```python
from build123d import *

# Parameters (mm, degrees)
CROQUIS1_R              = 3.25
CROQUIS1_R_2            = 2.25
SALIENTE_EXTRUIR1_DEPTH = 10
SALIENTE_EXTRUIR2_DEPTH = 10
CROQUIS3_R              = 2.25
CORTAR_EXTRUIR1_DEPTH   = 128.867118525
CROQUIS4_R              = 10.9
CORTAR_EXTRUIR2_DEPTH   = 7
CROQUIS5_R              = 4.25
CORTAR_EXTRUIR3_DEPTH   = 128.667536986
CROQUIS6_R              = 2.5
CORTAR_EXTRUIR4_DEPTH   = 128.867118525


with BuildPart() as part:
    # Croquis1 → Saliente-Extruir1 (new body)
    with BuildSketch(Plane(origin=(0, 0, 0), x_dir=(0, 0, -1), z_dir=(1, 0, 0))):
        with BuildLine():
            Line((-25, 0), (-25, -85))
            Line((-25, -85), (25, -85))
            Line((25, -85), (25, 0))
            ThreePointArc((25, 0), (0, 25), (-25, 0))
        make_face()
        Circle(CROQUIS1_R, mode=Mode.SUBTRACT)
        with Locations((-8, 8)):
            Circle(CROQUIS1_R_2, mode=Mode.SUBTRACT)
        with Locations((8, 8)):
            Circle(CROQUIS1_R_2, mode=Mode.SUBTRACT)
        with Locations((8, -8)):
            Circle(CROQUIS1_R_2, mode=Mode.SUBTRACT)
        with Locations((-8, -8)):
            Circle(CROQUIS1_R_2, mode=Mode.SUBTRACT)
    extrude(amount=SALIENTE_EXTRUIR1_DEPTH)

    # Croquis2 → Saliente-Extruir2 (add)
    with BuildSketch(Plane(origin=(10, 0, 0), x_dir=(0, 0, -1), z_dir=(1, 0, 0))):
        with BuildLine():
            Line((-25, -100), (-25, -85))
            Line((-25, -85), (25, -85))
            Line((25, -85), (25, -100))
            ThreePointArc((25, -100), (0, -125), (-25, -100))
        make_face()
    extrude(amount=-SALIENTE_EXTRUIR2_DEPTH)

    # Croquis3 → Cortar-Extruir1 (cut, through all)
    with BuildSketch(Plane.ZY):
        with Locations((0, -35)):
            Circle(CROQUIS3_R)
        with Locations((0, -65)):
            Circle(CROQUIS3_R)
    extrude(amount=-CORTAR_EXTRUIR1_DEPTH, mode=Mode.SUBTRACT)

    # Croquis4 → Cortar-Extruir2 (cut)
    with BuildSketch(Plane.ZY):
        with Locations((0, -100)):
            Circle(CROQUIS4_R)
    extrude(amount=-CORTAR_EXTRUIR2_DEPTH, mode=Mode.SUBTRACT)

    # Croquis5 → Cortar-Extruir3 (cut, through all)
    with BuildSketch(Plane.ZY.offset(-7)):
        with Locations((0, -100)):
            Circle(CROQUIS5_R)
    extrude(amount=-CORTAR_EXTRUIR3_DEPTH, mode=Mode.SUBTRACT)

    # Croquis6 → Cortar-Extruir4 (cut, through all)
    with BuildSketch(Plane.ZY):
        with Locations((17.95, -100)):
            Circle(CROQUIS6_R)
    extrude(amount=-CORTAR_EXTRUIR4_DEPTH, mode=Mode.SUBTRACT)


solid = part.part
```
Source: CAD feature listing. Evaluate the final solid. Frame: model axes, mm. A direction names the side the tool comes from. Give positions to 0.01 mm unless a question says otherwise; leave off trailing zeros. Order: outer loops, then holes, each group sorted by start corner. A loop starts at its lowest first (then second) coordinate and runs counter-clockwise, first axis right, second up. Notation, with made-up numbers: (36, -4) -> (90, -4) arc R12 ccw to (90, 2) -> close; hole circle Ø2 at (63.5, 58). An arc over 180 degrees is marked (long way). Use a Markdown table: item, result.
Q1. Section D-D (z = 17.95). Return the cut outline in (x, y).
A:
| item | result |
|---|---|
| outline | (0, -117.4) -> (10, -117.4) -> (10, -102.5) -> (0, -102.5) -> close; (0, -97.5) -> (10, -97.5) -> (10, 17.4) -> (0, 17.4) -> close |
Q2. Pull-direction query (Y, two-part tool) for faces 3 (the face through (8.48, -103.77, 1.96)), 4 (the face through (5, -49, -25)), 5 (the face through (4.93, 24.994, -0.55)); classes: +Y half, -Y half, draft (parallel to the pull), parting line (faces both ways), or undercut.
A:
| item | result |
|---|---|
| face 3 | undercut |
| face 4 | draft |
| face 5 | +Y half |
Q3. Material intervals for line 1 (Y direction, x = 5.5, z = 0); line 2 (Z direction, x = 9, y = -99); line 3 (Y direction, x = 5.5, z = 2), sorted ascending. Write a range as [from, to].
A:
| item | result |
|---|---|
| line 1 | [-125, -110.9], [-89.1, -67.25], [-62.75, -37.25], [-32.75, -3.25], [3.25, 25] |
| line 2 | [-25, -4.13], [4.13, 15.66], [20.24, 25] |
| line 3 | [-124.92, -110.71], [-89.29, -66.03], [-63.97, -36.03], [-33.97, -2.56], [2.56, 24.92] |
Q4. Section A-A (z = 0). Return the cut outline in (x, y), and give its area (3 significant figures).
A:
| item | result |
|---|---|
| outline | (0, -125) -> (10, -125) -> (10, -104.25) -> (7, -104.25) -> (7, -110.9) -> (0, -110.9) -> close; (0, -89.1) -> (7, -89.1) -> (7, -95.75) -> (10, -95.75) -> (10, -67.25) -> (0, -67.25) -> close; (0, -62.75) -> (10, -62.75) -> (10, -37.25) -> (0, -37.25) -> close; (0, -32.75) -> (10, -32.75) -> (10, -3.25) -> (0, -3.25) -> close; (0, 3.25) -> (10, 3.25) -> (10, 25) -> (0, 25) -> close |
| area | 1,170 mm^2 |
Q5. First-contact query: P1, Ø19.5, axis at y = -100, z = 0, coming from the -X side; P2, Ø4, axis at y = 8, z = -8, coming from the -X side; P3, Ø1.5, axis at x = 4, z = 12, coming from the -Y side. Flat tips, straight axial feed; report the tip coordinate or a pass-through.
A:
| item | result |
|---|---|
| P1 | x = 7 |
| P2 | through |
| P3 | y = -122.33 |
Q6. Section B-B (y = -35). Return the cut outline in (x, z), and give its area (3 significant figures).
A:
| item | result |
|---|---|
| outline | (0, -25) -> (10, -25) -> (10, -2.25) -> (0, -2.25) -> close; (0, 2.25) -> (10, 2.25) -> (10, 25) -> (0, 25) -> close |
| area | 455 mm^2 |
Q7. Section C-C (x = 3.25). State how many separate pieces and enclosed holes the cut face has, and give its area (3 significant figures).
A:
| item | result |
|---|---|
| separate pieces | 1 |
| enclosed holes | 9 |
| area | 6,440 mm^2 |
Q8. Access query for faces 1 (the face through (5, -51, 25)), 2 (the face through (7, -105, 0)). Directions: +Z, -Z, +X, -X, +Y, -Y. A direction counts if a zero-diameter tool reaches every point of the face in a straight line with its end or side. Return the directions, or none.
A:
| item | result |
|---|---|
| face 1 | +Z, +X, -X, +Y, -Y |
| face 2 | -X |
